The drawing under review shows one solid part. Ordinate dimensions are in mm from its lowest x, y, z. Round coordinates to 2 decimals unless told otherwise and drop trailing zeros. Order: outer loops, then holes, each group sorted by start corner. A loop starts at its lowest first (then second) coordinate and runs counter-clockwise, first axis right, second up.
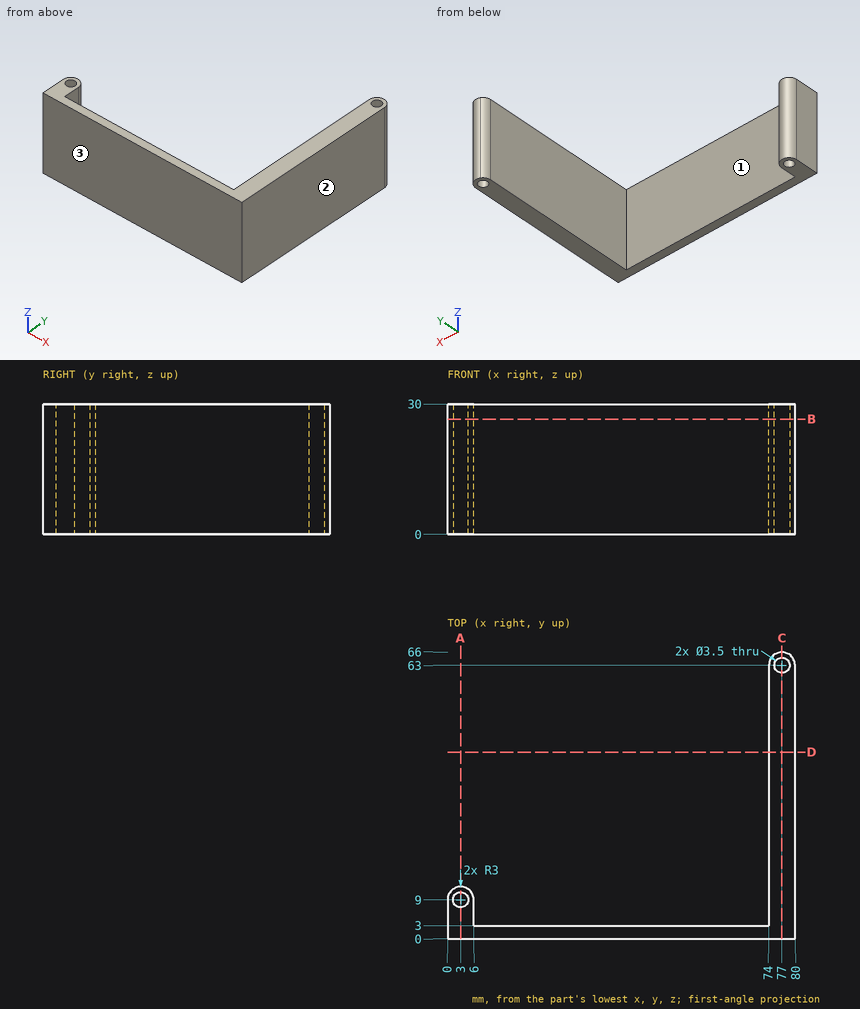
Q1. Take a section at B-B, the plane z = 26.5. State the section outline as (x, y) points, plus the area to 3 significant figures.
Q2. Take a section at A-A, the plane x = 3. State the section outline as (y, z) points, plus the area to 3 significant figures.
Q3. Take a section at D-D, the plane y = 43. State the section outline as (x, z) points, plus the area to 3 significant figures.
Q4. Take a section at C-C, the plane x = 77. State the section outline as (y, z) points, plus the area to 4 significant figures.
Q5. Wall thickness on line 1 (X direction, y = 9, z = 14.5); line 2 (Y direction, x = 3, z = 22.75); line 3 (X direction, y = 15.5, z = 23.5): over which ranges is each line inside the solid? List them lowest first.
Q6. Mouldability with a two-part tool opening along X and no side actions: class the marked faces 1, 2 and 3 as +X half, -X half, draft (parallel to the pull), parting line (faces both ways), or undercut.
Q7. Clearance check with flat-ended pins moving along their axes: pin 1 (1 mm diameter, centred on x = 57, z = 23, fed in from +Y); pin 2 (4 mm diameter, centred on y = 52, z = 9.5, fed in from -X); pin 3 (3 mm diameter, centred on x = 77, y = 63, fed in from +Z). State where each tip first meets the part, or that it passes through.
Working result:
1. outline: (0, 0) - (80, 0) - (80, 63) arc R3 ccw to (74, 63) - (74, 3) - (6, 3) - (6, 9) arc R3 ccw to (0, 9) - close; hole circle Ø3.5 at (3, 9); hole circle Ø3.5 at (77, 63)
1. area: 645 mm2
2. outline: (0, 0) - (7.25, 0) - (7.25, 30) - (0, 30) - close; (10.75, 0) - (12, 0) - (12, 30) - (10.75, 30) - close
2. area: 255 mm2
3. outline: (74, 0) - (80, 0) - (80, 30) - (74, 30) - close
3. area: 180 mm2
4. outline: (0, 0) - (61.25, 0) - (61.25, 30) - (0, 30) - close; (64.75, 0) - (66, 0) - (66, 30) - (64.75, 30) - close
4. area: 1,875 mm2
5. line 1: x = 0 to 1.25, 4.75 to 6, 74 to 80
5. line 2: y = 0 to 7.25, 10.75 to 12
5. line 3: x = 74 to 80
6. face 1: undercut
6. face 2: +X half
6. face 3: draft
7. pin 1: stops at y = 3
7. pin 2: stops at x = 74
7. pin 3: passes through
